The model under review builds one solid part; all positions refer to its coordinate system, in mm. A direction names the side the tool comes from. Round coordinates to 2 decimals unless told otherwise and drop trailing zeros. Write each loop counter-clockwise with the first axis right and the second up, starting at its lowest first coordinate (ties: lowest second). Pieces come first, ordered by that corner, then holes. Notation, with made-up numbers: (-29.5, 2) - (27.5, 2) arc R26 ccw to (27.5, 32) - close; hole circle Ø8 at (53.5, 45). An arc over 180 degrees is marked (long way). Return JSON: item names as keys, results as strings.
from build123d import *

# Parameters (mm, degrees)
SKETCH1_R                = 45.5
SKETCH1_R_2              = 33.5
BOSS_EXTRUDE1_DEPTH      = 4
SKETCH2_R                = 45.5
SKETCH2_R_2              = 37.5
BOSS_EXTRUDE2_DEPTH      = 83.3
SKETCH4_R                = 2
CUT_EXTRUDE1_DEPTH       = 6
CIRPATTERN1_COUNT        = 3
BOSS_EXTRUDE4_REACH      = 136.062
BOSS_EXTRUDE4_END_RADIUS = 45.5
SKETCH7_W                = 27.5
SKETCH7_H                = 47
SKETCH9_R                = 2
CUT_EXTRUDE2_DEPTH       = 6
SKETCH10_R               = 2
CUT_EXTRUDE3_DEPTH       = 6


with BuildPart() as part:
    # Sketch1 → Boss-Extrude1 (new body)
    with BuildSketch(Plane(origin=(0, 0, 0), x_dir=(1, 0, 0), z_dir=(0, 1, 0))):
        with Locations(Location((0, 0, 0), (0, 0, 270))):
            Circle(SKETCH1_R)
        with Locations(Location((0, 0, 0), (0, 0, 270))):
            Circle(SKETCH1_R_2, mode=Mode.SUBTRACT)
    extrude(amount=BOSS_EXTRUDE1_DEPTH)

    # Sketch2 → Boss-Extrude2 (add)
    with BuildSketch(Plane(origin=(0, 4, 0), x_dir=(1, 0, 0), z_dir=(0, 1, 0))):
        with Locations(Location((0, 0, 0), (0, 0, 270))):
            Circle(SKETCH2_R)
        with Locations(Location((0, 0, 0), (0, 0, 270))):
            Circle(SKETCH2_R_2, mode=Mode.SUBTRACT)
    extrude(amount=BOSS_EXTRUDE2_DEPTH)

    # Sketch4 → Cut-Extrude1 (cut)
    with BuildSketch(Plane(origin=(0, 87.3, 0), x_dir=(1, 0, 0), z_dir=(0, 1, 0))):
        with Locations(Location((0, 41.5, 0), (0, 0, 270))):
            Circle(SKETCH4_R)
    cut_extrude1 = extrude(amount=-CUT_EXTRUDE1_DEPTH, mode=Mode.SUBTRACT)

    # CirPattern1: Cut-Extrude1 ×3 about axis
    cirpattern1_axis = Axis((0, 0, 0), (0, 1, 0))
    for i in range(1, CIRPATTERN1_COUNT):
        add(cut_extrude1.rotate(cirpattern1_axis, i * 360 / CIRPATTERN1_COUNT), mode=Mode.SUBTRACT)

    # Boss-Extrude4: up to this cylinder (the profile starts outside it)
    boss_extrude4_end = Plane(origin=(0, 23.5, 0), z_dir=(0, -1, 0)) * Cylinder(BOSS_EXTRUDE4_END_RADIUS, 364.124, mode=Mode.PRIVATE)
    # Sketch7 → Boss-Extrude4 (add, up to the surface)
    with BuildSketch(Plane(origin=(0, 87.3, 45.5), x_dir=(1, 0, 0), z_dir=(0, 0, 1)), mode=Mode.PRIVATE) as boss_extrude4_sk1:
        with Locations((0, -63.8)):
            Rectangle(SKETCH7_W, SKETCH7_H)
    boss_extrude4_tool1 = extrude(boss_extrude4_sk1.sketch, amount=-BOSS_EXTRUDE4_REACH, mode=Mode.PRIVATE) - boss_extrude4_end
    add(boss_extrude4_tool1.solids().sort_by_distance((0, 23.5, 45.5))[0])
    add(boss_extrude4_tool1.solids().sort_by_distance((0, 23.5, 45.5))[1])

    # Sketch9 → Cut-Extrude2 (cut)
    with BuildSketch(Plane.XY.offset(45.5)):
        with Locations((-9.75, 4)):
            Circle(SKETCH9_R)
        with Locations((9.75, 4)):
            Circle(SKETCH9_R)
    extrude(amount=-CUT_EXTRUDE2_DEPTH, mode=Mode.SUBTRACT)

    # Sketch10 → Cut-Extrude3 (cut)
    with BuildSketch(Plane.XY.offset(45.5)):
        with Locations((-9.75, 43)):
            Circle(SKETCH10_R)
        with Locations((9.75, 43)):
            Circle(SKETCH10_R)
    extrude(amount=-CUT_EXTRUDE3_DEPTH, mode=Mode.SUBTRACT)


solid = part.part
(1) Add section A-A (z = 0). Write out the cut boundary in (x, y).
Filled in:
{"outline": "(-45.5, 0) - (-33.5, 0) - (-33.5, 4) - (-37.5, 4) - (-37.5, 87.3) - (-45.5, 87.3) - close; (33.5, 0) - (45.5, 0) - (45.5, 87.3) - (37.5, 87.3) - (37.5, 4) - (33.5, 4) - close"}
(2) Mouldability with a two-part tool opening along Z and no side actions: class faces 1 (the cylindrical face through (-27.686, 43.039, -36.107)), 2 (the cylindrical face through (9.316, 2.048, 42.542)), 3 (the flat face through (0, 81.3, -42)) as released by +Z, released by -Z, zero draft, split by the parting line, or undercut.
Filled in:
{"face 1": "split by the parting line", "face 2": "zero draft", "face 3": "undercut"}
(3) Add section C-C (x = 9.75). Write out the cut boundary in (y, z).
Filled in:
{"outline": "(0, -44.44) - (87.3, -44.44) - (87.3, -36.21) - (4, -36.21) - (4, -32.05) - (0, -32.05) - close; (0, 32.05) - (4, 32.05) - (4, 36.21) - (87.3, 36.21) - (87.3, 44.44) - (47, 44.44) - (47, 45.5) - (45, 45.5) - (45, 39.5) - (41, 39.5) - (41, 45.5) - (6, 45.5) - (6, 39.5) - (2, 39.5) - (2, 45.5) - (0, 45.5) - close"}
(4) Wall thickness on line 1 (Y direction, x = 9.75, z = 42.85); line 2 (X direction, y = 82, z = 20); line 3 (X direction, y = 75, z = -12): over which ranges is each line inside the solid? List them lowest first.
Filled in:
{"line 1": "y = 0 to 2, 6 to 41, 45 to 87.3", "line 2": "x = -40.87 to -37.79, -34.09 to -31.72, 31.72 to 34.09, 37.79 to 40.87", "line 3": "x = -43.89 to -35.53, 35.53 to 43.89"}
(5) Add section B-B (y = 43). Write out the cut boundary in (x, z), plus the area to 3 significant figures.
Filled in:
{"outline": "(-13.75, 43.37) arc R45.5 ccw (long way) to (13.75, 43.37) - (13.75, 45.5) - (11.75, 45.5) - (11.75, 39.5) - (7.75, 39.5) - (7.75, 45.5) - (-7.75, 45.5) - (-7.75, 39.5) - (-11.75, 39.5) - (-11.75, 45.5) - (-13.75, 45.5) - close; hole circle Ø75 at (0, 0)", "area": "2,060 mm2"}
(6) Clearance check with flat-ended pins moving along their axes: pin 1 Ø10 at (y, z) = (74, 36) entering from -X; pin 2 Ø3.5 at (x, z) = (-35.94, 20.75) entering from +Y; pin 3 Ø3 at (x, y) = (-9.5, 42.5) entering from +Z; pin 4 Ø5 at (x, y) = (-24, 13) entering from -Z. State where each tip first meets the part, or that it passes through.
Filled in:
{"pin 1": "stops at x = -33.31", "pin 2": "stops at y = 81.3", "pin 3": "stops at z = 45.5", "pin 4": "stops at z = -40.1"}
(7) For faces 4 (the flat face through (34, 87.3, -17)), 5 (the flat face through (-36, 81.3, 21)), 6 (the flat face through (-10, 4, 39.5)), list the 3-axis set-ups (+Z, -Z, +X, -X, +Y, -Y) from which the entire face can be reached by the end or side of a thin tool; tool diameter is ignored.
Filled in:
{"face 4": "+Z, -Z, +X, -X, +Y", "face 5": "+Y", "face 6": "+Z"}
(8) Add section D-D (z = 35). Write out the cut boundary in (x, y), plus the area to 3 significant figures.
Filled in:
{"outline": "(-29.07, 0) - (29.07, 0) - (29.07, 87.3) - (13.46, 87.3) - (13.46, 4) - (-13.46, 4) - (-13.46, 87.3) - (-29.07, 87.3) - close", "area": "2,830 mm2"}
